Here's how the part is built. I have some questions about the finished solid (model axes, mm). A direction names the side the tool comes from. Round coordinates to 2 decimals unless told otherwise and drop trailing zeros. Order: outer loops, then holes, each group sorted by start corner. A loop starts at its lowest first (then second) coordinate and runs counter-clockwise, first axis right, second up.
```python
from build123d import *

# Parameters (mm, degrees)
SKETCH1_R                = 100
BOSS_EXTRUDE1_DEPTH      = 5
BOSS_EXTRUDE2_START      = 16
SKETCH1_3_R              = 12.65
SKETCH1_3_W              = 7.4
SKETCH1_3_H              = 3.5
BOSS_EXTRUDE2_DEPTH      = 16
CHAMFER1_SIZE            = 14
CUT_EXTRUDE1_DEPTH       = 146.988090268
CUT_EXTRUDE1_DEPTH_BACK  = 5.15
SKETCH3_R                = 2
FILLET1_R                = 3
BOSS_EXTRUDE3_START      = 60
BOSS_EXTRUDE3_DEPTH      = 60
FILLET3_R                = 8
FILLET4_R                = 8
CIRPATTERN1_COUNT        = 8
FILLET3_OF_CIRPATTERN1_R = 8
FILLET4_OF_CIRPATTERN1_R = 8


with BuildPart() as part:
    # Sketch1 → Boss-Extrude1 (new body)
    with BuildSketch(Plane(origin=(0, 0, 0), x_dir=(1, 0, 0), z_dir=(0, 1, 0))):
        with Locations(Location((0, 0, 0), (0, 0, 270))):
            Circle(SKETCH1_R)
        with BuildLine():
            Line((2.549509757, -1.85), (-2.549509757, -1.85))
            ThreePointArc((-2.549509757, -1.85), (0, 3.15), (2.549509757, -1.85))
        make_face(mode=Mode.SUBTRACT)
    extrude(amount=-BOSS_EXTRUDE1_DEPTH)

    # Sketch1<3> → Boss-Extrude2 (add)
    with BuildSketch(Plane(origin=(0, 0, 0), x_dir=(1, 0, 0), z_dir=(0, 1, 0)).offset(BOSS_EXTRUDE2_START)):
        with Locations(Location((0, 0, 0), (0, 0, 270))):
            Circle(SKETCH1_3_R)
        with BuildLine():
            Line((2.549509757, -1.85), (-2.549509757, -1.85))
            ThreePointArc((-2.549509757, -1.85), (0, 3.15), (2.549509757, -1.85))
        make_face(mode=Mode.SUBTRACT)
        with Locations((0, -6.9)):
            Rectangle(SKETCH1_3_W, SKETCH1_3_H, mode=Mode.SUBTRACT)
    extrude(amount=-BOSS_EXTRUDE2_DEPTH)

    # Chamfer1
    chamfer1_edges = [part.edges().sort_by_distance(p)[0] for p in [
        (0, 0, -12.65),
    ]]
    chamfer(chamfer1_edges, length=CHAMFER1_SIZE)

    # Sketch3 → Cut-Extrude1 (cut, two sides: drawn at the far end of the back side and taken through both)
    with BuildSketch(Plane.XY.offset(5.15).offset(-CUT_EXTRUDE1_DEPTH_BACK)):
        with Locations(Location((0, 8, 0), (0, 0, 180))):
            Circle(SKETCH3_R)
    extrude(amount=CUT_EXTRUDE1_DEPTH + CUT_EXTRUDE1_DEPTH_BACK, mode=Mode.SUBTRACT)

    # Fillet1
    fillet1_edges = [part.edges().sort_by_distance(p)[0] for p in [
        (3.7, 0, 6.9),
        (-3.7, 0, 6.9),
    ]]
    fillet(fillet1_edges, radius=FILLET1_R)

    # Sketch4 → Boss-Extrude3 (add)
    with BuildSketch(Plane(origin=(0, 0, 0), x_dir=(1, 0, 0), z_dir=(0, 1, 0)).offset(BOSS_EXTRUDE3_START)):
        with BuildLine():
            Line((-22.374700612, -44.714346384), (-30, -40))
            ThreePointArc((-30, -40), (-24.010405369, -74.505202685), (0, -100))
            ThreePointArc((0, -100), (8.67647844, -99.622882521), (17.287515846, -98.494374438))
            ThreePointArc((17.287515846, -98.494374438), (-12.116392899, -78.664202138), (-22.374700612, -44.714346384))
        make_face()
    boss_extrude3 = extrude(amount=-BOSS_EXTRUDE3_DEPTH)

    # Fillet3
    fillet3_edges = [part.edges().sort_by_distance(p)[0] for p in [
        (-22.374700612, 30, 44.714346384),
    ]]
    fillet(fillet3_edges, radius=FILLET3_R)

    # Fillet4
    # the kernel refuses this fillet: 8 mm, written as the material it takes off along each edge
    with BuildSketch(Plane(origin=(0, 66.107971256, 100), x_dir=(0.999929553100501, 0, -0.01186966032505709), z_dir=(0, -1, 0))) as fillet4_piece_1:
        with BuildLine():
            CenterArc((2.278974782, -7.999436425), FILLET4_R, 89.319902589, 33.659920931)
            ThreePointArc((-2.075774552, -1.288537958), (-1.044352376, -0.633854003), (0, 0))
            ThreePointArc((0, 0), (1.186966033, 0.00704469), (2.373932065, 0))
        make_face()
    extrude(amount=66.107971256, mode=Mode.SUBTRACT)

    # CirPattern1: Boss-Extrude3 ×8 about axis
    cirpattern1_axis = Axis((0, 0, 0), (0, 1, 0))
    for i in range(1, CIRPATTERN1_COUNT):
        add(boss_extrude3.rotate(cirpattern1_axis, i * 360 / CIRPATTERN1_COUNT))

    # Fillet3 of CirPattern1
    fillet3_of_cirpattern1_edges = [part.edges().sort_by_distance(p)[0] for p in [
        (15.796515014, 30, 47.439120074),
        (44.714346384, 30, 22.374700612),
        (47.439120074, 30, -15.796515014),
        (22.374700612, 30, -44.714346384),
        (-15.796515014, 30, -47.439120074),
        (-44.714346384, 30, -22.374700612),
        (-47.439120074, 30, 15.796515014),
    ]]
    fillet(fillet3_of_cirpattern1_edges, radius=FILLET3_OF_CIRPATTERN1_R)

    # Fillet4 of CirPattern1
    # the kernel refuses this fillet: 8 mm, written as the material it takes off along each edge
    with BuildSketch(Plane(origin=(70.710678119, 66.107971256, 70.710678119), x_dir=(0.6986638503999697, 0, -0.7154500850124269), z_dir=(0, -1, 0)), Plane(origin=(100, 66.107971256, 0), x_dir=(-0.01186966032505703, 0, -0.9999295531005011), z_dir=(0, -1, 0)), Plane(origin=(70.710678119, 66.107971256, -70.710678119), x_dir=(-0.7154500850124297, 0, -0.6986638503999666), z_dir=(0, -1, 0)), Plane(origin=(0, 66.107971256, -100), x_dir=(-0.999929553100501, 0, 0.011869660325056916), z_dir=(0, -1, 0))) as fillet4_of_cirpattern1_piece_1:
        with BuildLine():
            CenterArc((2.278974782, -7.999436425), FILLET4_OF_CIRPATTERN1_R, 89.319902589, 33.659920931)
            ThreePointArc((-2.075774552, -1.288537958), (-1.044352376, -0.633854003), (0, 0))
            ThreePointArc((0, 0), (1.186966033, 0.00704469), (2.373932065, 0))
        make_face()
    extrude(amount=66.107971256, mode=Mode.SUBTRACT)
    with BuildSketch(Plane(origin=(-70.710678119, 66.107971256, -70.710678119), x_dir=(0.9709251782861501, 0, -0.23938316183476163), z_dir=(0, -1, 0)), Plane(origin=(-100, 66.107971256, 0), x_dir=(0.517278320555659, 0, -0.8558172346261301), z_dir=(0, -1, 0)), Plane(origin=(-70.710678119, 66.107971256, 70.710678119), x_dir=(-0.23938316183476574, 0, -0.9709251782861491), z_dir=(0, -1, 0))) as fillet4_of_cirpattern1_piece_2:
        with BuildLine():
            CenterArc((2.282648109, 7.998389012), FILLET4_OF_CIRPATTERN1_R, 237.489942123, 33.659920931)
            ThreePointArc((-2.016933103, 1.252012103), (-1.012181922, 0.620020763), (0, 0))
            ThreePointArc((0, 0), (1.221594251, -0.012258436), (2.443188502, 0))
        make_face()
    extrude(amount=66.107971256, mode=Mode.SUBTRACT)


solid = part.part
```
1. If we section it at A-A, the plane y = 46: State how many separate pieces and enclosed holes the cut face has, and give its area (3 significant figures).
Evaluation:
separate pieces: 8
enclosed holes: 0
area: 4,550 mm2
2. On a 3-axis mill with a long thin cutter (end or side, diameter ignored), from which of +Z, -Z, +X, -X, +Y, -Y can I reach the whole of each face in a straight line? I mean faces 1 (the cylindrical face through (-10.539, 30.42, 80.698)), 2 (the cylindrical face through (-0.1, 5.65, -3.15)). Say none if no direction works.
Evaluation:
face 1: +Y
face 2: +Y, -Y
3. I'm going to push flat-ended pins straight in: P1, Ø3.5, axis at x = 0, y = 8, coming from the -Z side; P2, Ø1.5, axis at y = 4, z = 70, coming from the +X side; P3, Ø3, axis at x = -65.5, y = 31, coming from the -Z side. Where does each tip first touch, or does it pass through?
Evaluation:
P1: stops at z = -99.96
P2: stops at x = 72.13
P3: stops at z = -72.11
4. I need wall thicknesses on probe 1 along Z at (x, y) = (-68.5, 55.5); probe 2 along X at (y, z) = (11, 68); probe 3 along Z at (x, y) = (0, 3). Which ranges of each line are inside material? Lowest first, please.
Evaluation:
probe 1: z = -71.26 to -63.02, -26.62 to -17.99, 32.52 to 72.85
probe 2: x = -71.37 to -63.15, -26.8 to -18.21, 31.3 to 73.32
probe 3: z = -99.67 to -90.52, -23.65 to -3.15, 1.85 to 5.15, 8.65 to 23.65, 90.52 to 99.67
5. If we section it at B-B, the plane x = -78: Write out the boundary of the cut face in (y, z), and give its area (3 significant figures).
Evaluation:
outline: (-5, -62.58) - (60, -62.58) - (60, -59.5) - (0, -59.5) - (0, -22.12) - (60, -22.12) - (60, -12.6) - (0, -12.6) - (0, 62.58) - (-5, 62.58) - close
area: 1,380 mm2
6. If we mould it in two halves opening along Z, with no side actions, what happens to faces 3 (the cylindrical face through (23.454, 29.58, -45.199)), 4 (the cylindrical face through (0.082, 30.42, 99.693))? For each: released by +Z, released by -Z, zero draft, split by the parting line, or undercut.
Evaluation:
face 3: undercut
face 4: released by +Z
